Part model, mm, in its own coordinate system. A direction names the side the tool comes from. Round coordinates to 2 decimals unless told otherwise and drop trailing zeros. Write each loop counter-clockwise with the first axis right and the second up, starting at its lowest first coordinate (ties: lowest second). Pieces come first, ordered by that corner, then holes. Notation, with made-up numbers: M 66.5,51.5 L 103.5,51.5 A30 cw 103.5,84.5 Z; hole C -31.5,75.5 d4. An arc over 180 degrees is marked long. Use one line per item in the form item = value. Start each with the question number.
Item 1: Flat gauge pins, fed straight in: pin 1 Ø2 at (x, z) = (31, 24.5) entering from -Y; pin 2 Ø4 at (x, y) = (21.59, 9.525) entering from +Z; pin 3 Ø5 at (x, y) = (-21.59, 9.525) entering from +Z; pin 4 Ø5 at (x, y) = (21.59, 9.525) entering from -Z. Where does each tip first touch, or does it go through?
Item 2: Cut at C-C, the plane y = 2.5. Give the cut face in (x, z) (3 decimals), then the cut area to 3 significant figures.
Item 3: Probe L1, parallel to X at y = 12.75, z = -95.25 (3 decimals); L2, parallel to Z at x = 21.59, y = 15 (3 decimals); L3, parallel to X at y = 9.75, z = 88.5. List the from-to ranges inside material, lowest first.
Item 4: Cut at A-A, the plane z = 95.25. Give the cut face in (x, y) (3 decimals).
Item 5: Which spindle directions (+Z, -Z, +X, -X, +Y, -Y) get a long thin tool onto all of the face, cutting with end or side? Do faces 1 (the face through (20.636, 12.553, -109.336)), 2 (the face through (-46.99, 9, 2)), 3 (the face through (-20.636, 12.553, 109.336)). Say none if no direction does.
Item 6: Mould opens along Z. For faces 4 (the face through (24.451, 9.658, -86.165)), 5 (the face through (-24.451, 9.658, -86.165)), 6 (the face through (-1, 19.05, -2)), 7 (the face through (-1, 9, 114.3)) say: +Z half, -Z half, draft (parallel to the pull), parting line (faces both ways), or undercut.
Item 7: Cut at B-B, the plane x = 21.59. Give the cut face in (y, z) (3 decimals).
from build123d import *

# Parameters (mm, degrees)
SKETCH1_W           = 93.98
SKETCH1_H           = 228.6
BOSS_EXTRUDE1_DEPTH = 19.05


with BuildPart() as part:
    # Sketch1 → Boss-Extrude1 (new body)
    with BuildSketch(Plane(origin=(0, 0, 0), x_dir=(1, 0, 0), z_dir=(0, 1, 0))):
        Rectangle(SKETCH1_W, SKETCH1_H)
    extrude(amount=BOSS_EXTRUDE1_DEPTH)

    # Sketch2 → 3/4 (0.75) Diameter Hole1 (revolve, cut)
    with BuildSketch(Plane(origin=(-21.59, 19.05, -95.25), x_dir=(0, 0, 1), z_dir=(1, 0, 0))):
        Polygon((0, 0), (0, 24.773197396), (9.525, 19.05), (9.525, 0), align=None)
    f_3_4_0_75_diameter_hole1 = revolve(axis=Axis((-21.59, 25.4, -95.25), (0, -1, 0)), mode=Mode.SUBTRACT)

    # Mirror1: 3/4 (0.75) Diameter Hole1 across plane
    add(f_3_4_0_75_diameter_hole1.mirror(Plane.XY), mode=Mode.SUBTRACT)

    # Mirror4: 3/4 (0.75) Diameter Hole1 across plane
    add(f_3_4_0_75_diameter_hole1.mirror(Plane(origin=(0, 0, 0), x_dir=(0, 0, 1), z_dir=(1, 0, 0))), mode=Mode.SUBTRACT)

    # Mirror4 copy 1 sketch → Mirror4 copy 1 (revolve, cut)
    with BuildSketch(Plane(origin=(21.59, 19.05, 95.25), x_dir=(0, 0, -1), z_dir=(-1, 0, 0))):
        Polygon((0, 0), (0, 24.773197396), (9.525, 19.05), (9.525, 0), align=None)
    revolve(axis=Axis((21.59, 25.4, 95.25), (0, -1, 0)), mode=Mode.SUBTRACT)

    # Sketch4 → 1/4 (0.25) Diameter Hole1 (revolve, cut)
    with BuildSketch(Plane(origin=(21.59, 9.525, -114.3), x_dir=(0, 1, 0), z_dir=(1, 0, 0))):
        Polygon((0, 0), (0, 20.957732465), (3.175, 19.05), (3.175, 0), align=None)
    f_1_4_0_25_diameter_hole1 = revolve(axis=Axis((21.59, 9.525, -120.65), (0, 0, 1)), mode=Mode.SUBTRACT)

    # Mirror5: 1/4 (0.25) Diameter Hole1 across plane
    add(f_1_4_0_25_diameter_hole1.mirror(Plane.XY), mode=Mode.SUBTRACT)

    # Mirror10: 1/4 (0.25) Diameter Hole1 across plane
    add(f_1_4_0_25_diameter_hole1.mirror(Plane(origin=(0, 0, 0), x_dir=(0, 0, 1), z_dir=(1, 0, 0))), mode=Mode.SUBTRACT)

    # Mirror10 copy 1 sketch → Mirror10 copy 1 (revolve, cut)
    with BuildSketch(Plane(origin=(-21.59, 9.525, 114.3), x_dir=(0, 1, 0), z_dir=(-1, 0, 0))):
        Polygon((0, 0), (0, 20.957732465), (3.175, 19.05), (3.175, 0), align=None)
    revolve(axis=Axis((-21.59, 9.525, 120.65), (0, 0, -1)), mode=Mode.SUBTRACT)


solid = part.part
Model answer:
q1.pin_1 = 0
q1.pin_2 = 85.94
q1.pin_3 = 86.06
q1.pin_4 = -86.06
q2.outline = M -46.99,-114.3 L 46.99,-114.3 L 46.99,114.3 L -46.99,114.3 Z; hole C -21.59,-95.25 d19.05; hole C -21.59,95.25 d19.05; hole C 21.59,-95.25 d19.05; hole C 21.59,95.25 d19.05
q2.area = 20,300 mm²
q3.L1 = -46.99 to -31.115, -12.065 to 12.065, 31.115 to 46.99
q3.L2 = -114.3 to -104.775, -85.725 to 85.725, 104.775 to 114.3
q3.L3 = -46.99 to -28.31, -14.87 to 14.87, 28.31 to 46.99
q4.outline = M -46.99,0 L -31.115,0 L -31.115,19.05 L -46.99,19.05 Z; M -12.065,0 L 12.065,0 L 12.065,19.05 L -12.065,19.05 Z; M 31.115,0 L 46.99,0 L 46.99,19.05 L 31.115,19.05 Z
q5.face_1 = -Z
q5.face_2 = +Z, -Z, -X, +Y, -Y
q5.face_3 = +Z
q6.face_4 = undercut
q6.face_5 = undercut
q6.face_6 = draft
q6.face_7 = +Z half
q7.outline = M 0,-114.3 L 6.35,-114.3 L 6.35,-104.775 L 0,-104.775 Z; M 0,-85.725 L 19.05,-85.725 L 19.05,85.725 L 0,85.725 Z; M 0,104.775 L 6.35,104.775 L 6.35,114.3 L 0,114.3 Z; M 12.7,-114.3 L 19.05,-114.3 L 19.05,-104.775 L 12.7,-104.775 Z; M 12.7,104.775 L 19.05,104.775 L 19.05,114.3 L 12.7,114.3 Z
